```python
from build123d import *

# Parameters (mm, degrees)
BOSS_EXTRUDE1_DEPTH     = 7.5
CUT_EXTRUDE1_DEPTH      = 5
CUT_EXTRUDE1_DEPTH_BACK = 25
SKETCH3_W               = 11
SKETCH3_H               = 65
SKETCH5_R               = 2.5
BOSS_EXTRUDE3_DEPTH     = 11
SKETCH6_R               = 2.5
BOSS_EXTRUDE4_DEPTH     = 13
FILLET1_R               = 1
FILLET2_R               = 4.7
FILLET3_R               = 15.1
FILLET4_R               = 2.8
FILLET7_R               = 1
CUT_EXTRUDE2_START      = -1.5
CUT_EXTRUDE2_DEPTH      = 1.5


with BuildPart() as part:
    # Sketch1 → Boss-Extrude1 (new, symmetric)
    with BuildSketch(Plane.XY):
        with BuildLine():
            Line((5, 41.700950662), (6.5, 41.700950662))
            Line((6.5, 41.700950662), (6.5, -18.299049338))
            Line((6.5, -18.299049338), (-17, -18.299049338))
            Line((-17, -18.299049338), (-20.5, -8.299049338))
            Line((-20.5, -8.299049338), (-12.631273367, 1.700950662))
            Line((-12.631273367, 1.700950662), (-6.631273367, 1.700950662))
            ThreePointArc((-6.631273367, 1.700950662), (-7.739623811, 21.779414386), (-5, 41.700950662))
            ThreePointArc((-5, 41.700950662), (0, 46.700950662), (5, 41.700950662))
        make_face()
    extrude(amount=BOSS_EXTRUDE1_DEPTH, both=True)

    # Sketch3 → Cut-Extrude1 (cut, two sides: drawn at the far end of the back side and taken through both)
    with BuildSketch(Plane(origin=(0, 0, 0), x_dir=(0, 0, -1), z_dir=(1, 0, 0)).offset(-CUT_EXTRUDE1_DEPTH_BACK)):
        with Locations((0, 14.200950662)):
            Rectangle(SKETCH3_W, SKETCH3_H)
    extrude(amount=CUT_EXTRUDE1_DEPTH + CUT_EXTRUDE1_DEPTH_BACK, mode=Mode.SUBTRACT)

    # Sketch5 → Boss-Extrude3 (add)
    with BuildSketch(Plane.XY.offset(-5.5)):
        with Locations((0, 41.700950662)):
            Circle(SKETCH5_R)
    extrude(amount=BOSS_EXTRUDE3_DEPTH)

    # Sketch6 → Boss-Extrude4 (add)
    with BuildSketch(Plane.XY.offset(7.5)):
        with Locations(Location((0, -13.299049338, 0), (0, 0, 90))):
            Circle(SKETCH6_R)
    extrude(amount=-BOSS_EXTRUDE4_DEPTH)

    # Fillet1
    fillet1_edges = [part.edges().sort_by_distance(p)[0] for p in [
        (6.5, 11.700950662, 7.5),
        (6.5, 11.700950662, -7.5),
    ]]
    fillet(fillet1_edges, radius=FILLET1_R)

    # Fillet2
    fillet2_edges = [part.edges().sort_by_distance(p)[0] for p in [
        (-12.631273367, 1.700950662, 6.5),
        (-12.631273367, 1.700950662, -6.5),
    ]]
    fillet(fillet2_edges, radius=FILLET2_R)

    # Fillet3
    fillet3_edges = [part.edges().sort_by_distance(p)[0] for p in [
        (-20.5, -8.299049338, 6.5),
        (-20.5, -8.299049338, -6.5),
    ]]
    fillet(fillet3_edges, radius=FILLET3_R)

    # Fillet4
    fillet4_edges = [part.edges().sort_by_distance(p)[0] for p in [
        (-17, -18.299049338, 6.5),
        (-17, -18.299049338, -6.5),
    ]]
    fillet(fillet4_edges, radius=FILLET4_R)

    # Fillet7
    fillet7_edges = [part.edges().sort_by_distance(p)[0] for p in [
        (-4.756726593, -18.299049338, -7.5),
        (-4.756726593, -18.299049338, 7.5),
        (-16.633646488, -17.782681021, 7.5),
        (-16.633646488, -17.782681021, -7.5),
        (-8.490130072, 1.700950662, 7.5),
        (6.5, -18.299049338, 0),
        (6.207106781, -18.299049338, 7.207106781),
        (6.207106781, -18.299049338, -7.207106781),
        (-8.490130072, 1.700950662, -7.5),
        (-14.710530592, -0.941480981, 7.5),
        (-12.40202012, 1.22884069, 7.5),
        (-14.710530592, -0.941480981, -7.5),
        (-12.40202012, 1.22884069, -7.5),
        (-17.710124778, -16.2701214, 7.5),
        (-18.406636263, -8.647634431, 7.5),
        (-17.710124778, -16.2701214, -7.5),
        (-18.406636263, -8.647634431, -7.5),
    ]]
    fillet(fillet7_edges, radius=FILLET7_R)

    # Sketch7 → Cut-Extrude2 (cut)
    with BuildSketch(Plane(origin=(0, 41.700950662, 0), x_dir=(1, 0, 0), z_dir=(0, 1, 0)).offset(CUT_EXTRUDE2_START)):
        with BuildLine():
            Line((6.5, -6.5), (6.5, 6.5))
            ThreePointArc((6.5, 6.5), (6.207106781, 7.207106781), (5.5, 7.5))
            Line((5.5, 7.5), (5, 7.5))
            Line((5, 7.5), (5, 5.5))
            Line((5, 5.5), (5, -5.5))
            Line((5, -5.5), (5, -7.5))
            Line((5, -7.5), (5.5, -7.5))
            ThreePointArc((5.5, -7.5), (6.207106781, -7.207106781), (6.5, -6.5))
        make_face()
    extrude(amount=CUT_EXTRUDE2_DEPTH, mode=Mode.SUBTRACT)


solid = part.part
```
The model under review builds one solid part; all positions refer to its coordinate system, in mm. A direction names the side the tool comes from. Coordinates: 2 decimals unless noted, no trailing zeros. Order: outer loops, then holes, each group sorted by start corner. A loop starts at its lowest first (then second) coordinate and runs counter-clockwise, first axis right, second up. Notation, with made-up numbers: (60.5, -2) -> (90.5, -2) arc R17 cw to (90.5, 31) -> close; hole circle Ø1 at (32, -36). An arc over 180 degrees is marked (long way). Answer in a Markdown table with one row per item. Add a question column.
Item 1: Mouldability with a two-part tool opening along Y and no side actions: class faces 4 (the cylindrical face through (1.34, 43.81, -0.08)), 5 (the flat face through (-3, 8, -7.5)), 6 (the flat face through (-14.72, -0.953, 6.007)) as +Y half, -Y half, draft (parallel to the pull), parting line (faces both ways), or undercut.
Item 2: Clearance check with flat-ended pins moving along their axes: pin 1 (4 mm diameter, centred on x = -3.5, z = 0, fed in from -Y); pin 2 (1.2 mm diameter, centred on y = 41, z = 6.5, fed in from +X); pin 3 (0.8 mm diameter, centred on x = -9, z = -6, fed in from +Y). State where each tip first meets the part, or that it passes through.
Item 3: We need section A-A on z = 4. Write out the cut boundary in (x, y), plus the area to 3 significant figures.
Item 4: We need section D-D on y = 34.5. Write out the cut boundary in (x, z), plus the area to 3 significant figures.
Item 5: We need section B-B on x = -9. Write out the cut boundary in (y, z).
Item 6: Machinability: for faces 1 (the flat face through (5, 41, -7)), 2 (the cylindrical face through (-12.38, 1.24, 5.99)), 3 (the cylindrical face through (-0.751, -10.914, 0.077)), which of the approach directions +Z, -Z, +X, -X, +Y, -Y give a long, thin tool a straight path to every point of the face, cutting with its end or side? Answer none if there is none.
Item 7: We need section C-C on x = 0. Write out the cut boundary in (y, z), plus the area to 3 significant figures.
Item 8: To check wall thickness, follow probe 1 along Z at (x, y) = (1.75, 3.5); probe 2 along X at (y, z) = (27.5, -0.75); probe 3 along Y at (x, z) = (-1, 2). State the ranges of each line that lie inside material, in increasing order.
Final values:
| question | item | result |
|---|---|---|
| 1 | face 4 | undercut |
| 1 | face 5 | draft |
| 1 | face 6 | +Y half |
| 2 | pin 1 | stops at y = -15.3 |
| 2 | pin 2 | stops at x = 5 |
| 2 | pin 3 | stops at y = 1.7 |
| 3 | outline | circle Ø5 at (0, -13.3); circle Ø5 at (0, 41.7); (5, -18.3) -> (5.5, -18.3) arc R1 ccw to (6.5, -17.3) -> (6.5, 40.2) -> (5, 40.2) -> close |
| 3 | area | 127 mm2 |
| 4 | outline | (-6.44, -7.5) -> (5.5, -7.5) arc R1 ccw to (6.5, -6.5) -> (6.5, 6.5) arc R1 ccw to (5.5, 7.5) -> (-6.44, 7.5) -> (-6.44, 5.5) -> (5, 5.5) -> (5, -5.5) -> (-6.44, -5.5) -> close |
| 4 | area | 67.8 mm2 |
| 5 | outline | (-18.3, -6.5) arc R1 ccw to (-17.3, -7.5) -> (0.7, -7.5) arc R1 ccw to (1.7, -6.5) -> (1.7, -5.5) -> (-18.3, -5.5) -> close; (-18.3, 5.5) -> (1.7, 5.5) -> (1.7, 6.5) arc R1 ccw to (0.7, 7.5) -> (-17.3, 7.5) arc R1 ccw to (-18.3, 6.5) -> close |
| 6 | face 1 | +Z, -Z, +X, +Y |
| 6 | face 2 | +Z, -Z, -X, +Y |
| 6 | face 3 | none |
| 7 | outline | (-18.3, -6.5) arc R1 ccw to (-17.3, -7.5) -> (46.7, -7.5) -> (46.7, -5.5) -> (44.2, -5.5) -> (44.2, 5.5) -> (46.7, 5.5) -> (46.7, 7.5) -> (-17.3, 7.5) arc R1 ccw to (-18.3, 6.5) -> (-18.3, 5.5) -> (-15.8, 5.5) -> (-15.8, -5.5) -> (-18.3, -5.5) -> close; hole (-10.8, -5.5) -> (39.2, -5.5) -> (39.2, 5.5) -> (-10.8, 5.5) -> close |
| 7 | area | 370 mm2 |
| 8 | probe 1 | z = -7.5 to -5.5, 5.5 to 7.5 |
| 8 | probe 2 | x = 5 to 6.5 |
| 8 | probe 3 | y = -15.59 to -11.01, 39.41 to 43.99 |
